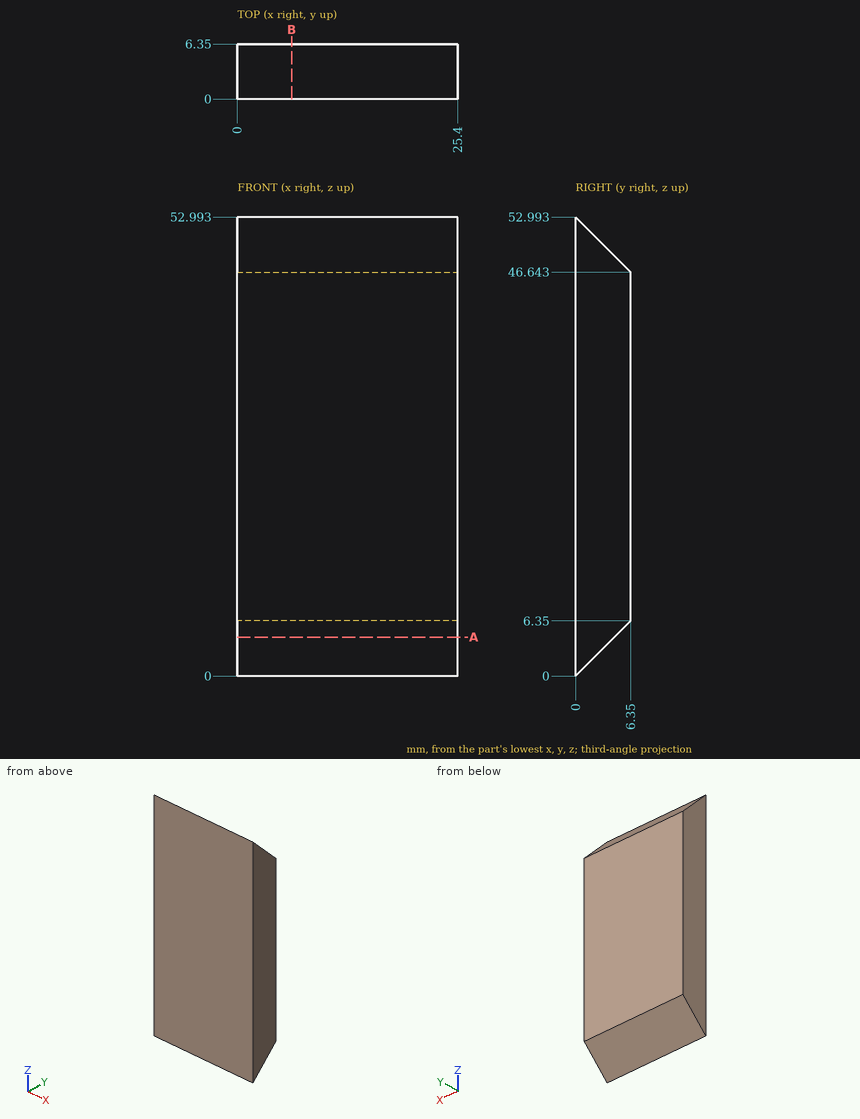
Could you check a few things on this drawing? It's one solid part, dimensions in mm from its lowest x, y, z. Round coordinates to 2 decimals unless told otherwise and drop trailing zeros. Write each loop counter-clockwise with the first axis right and the second up, starting at its lowest first coordinate (ties: lowest second). Pieces come first, ordered by that corner, then holes. Notation, with made-up numbers: (-24.5, -13.75) -> (4.5, -13.75) arc R12 cw to (4.5, -3.75) -> close; hole circle Ø5 at (-22, -7.75). An arc over 180 degrees is marked (long way). One line per question, with ' | ' between items. Start each with the question number.
1) Suppose I cut it at B-B on x = 6.25. Write out the boundary of the cut face in (y, z).
2) I need wall thicknesses on line 1 (Z direction, x = 17.5, y = 3.5) (1 decimal); line 2 (Z direction, x = 23, y = 2) (1 decimal); line 3 (Y direction, x = 4, z = 3). Which ranges of each line are inside material? Lowest first, please. Write a range as [from, to].
3) I'm going to push a flat-ended pin straight in: P1, Ø1.5, axis at x = 7, y = 3.5, coming from the -Z side. Where does the tip first touch, or does it pass through?
4) Suppose I cut it at A-A on z = 4.5. Write out the boundary of the cut face in (x, y).
Return value:
1) outline: (0, 0) -> (6.35, 6.35) -> (6.35, 46.64) -> (0, 52.99) -> close
2) line 1: z = [3.5, 49.5] | line 2: z = [2, 51] | line 3: y = [0, 3]
3) P1: stops at z = 2.75
4) outline: (0, 0) -> (25.4, 0) -> (25.4, 4.5) -> (0, 4.5) -> close
